Design review of the part shown in the three views and the two pictorial views. Dimensions are in mm from the part's minimum x, y and z. Give positions to 0.01 mm unless a question says otherwise; leave off trailing zeros. Write each loop counter-clockwise with the first axis right and the second up, starting at its lowest first coordinate (ties: lowest second). Pieces come first, ordered by that corner, then holes. Notation, with made-up numbers: (59, 65) -> (98, 65) arc R13 cw to (98, 81) -> close; hole circle Ø5 at (49.5, 64.25). An arc over 180 degrees is marked (long way). Return JSON: item names as keys, results as strings. Group by question number.
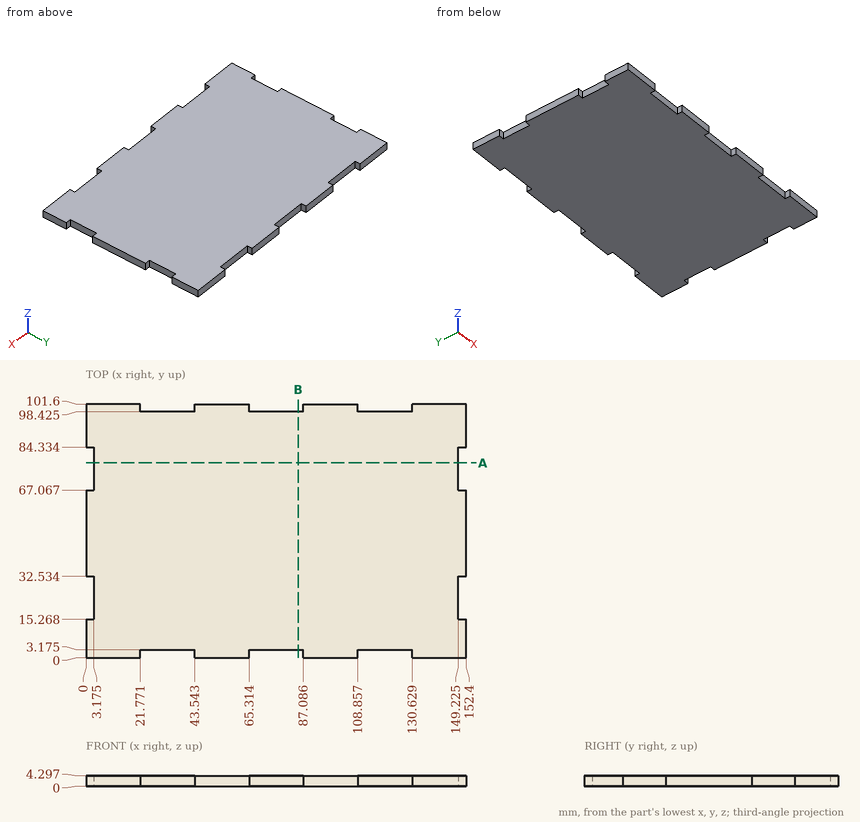
Q1. Insertion check: pin 1 (1 mm diameter, centred on x = 1, z = 3, fed in from -Y); pin 2 (2 mm diameter, centred on x = 30, z = 1.5, fed in from -Y) (3 decimals). Each pin has a flat end and moves straight along its axis. Give the tip position at first contact, or say it passes through.
Q2. For L1, parallel to Y at x = 126.5, z = 1.8 (1 decimal); L2, parallel to X at y = 79, z = 3.95 (1 decimal), list the stretches that pass through material, from the lowest coordinate up. Write a range as from..to.
Q3. Take a section at B-B, the plane x = 85. Give the boundary of the cut face in (y, z) (1 decimal).
Q4. Take a section at A-A, the plane y = 78. Give the boundary of the cut face in (x, z) (1 decimal).
Final values:
{
 "1": {"pin 1": "stops at y = 0", "pin 2": "stops at y = 3.175"},
 "2": {"L1": "y = 3.2..98.4", "L2": "x = 3.2..149.2"},
 "3": {"outline": "(3.2, 0) -> (98.4, 0) -> (98.4, 4.3) -> (3.2, 4.3) -> close"},
 "4": {"outline": "(3.2, 0) -> (149.2, 0) -> (149.2, 4.3) -> (3.2, 4.3) -> close"}
}
